Could you check a few things on this model? Use its own coordinates, in mm. A direction names the side the tool comes from. Give positions to 0.01 mm unless a question says otherwise; leave off trailing zeros. Write each loop counter-clockwise with the first axis right and the second up, starting at its lowest first coordinate (ties: lowest second). Pieces come first, ordered by that corner, then holes. Notation, with made-up numbers: (45.5, 45.25) - (74.5, 45.25) arc R23 ccw to (74.5, 61.25) - close; hole circle Ø7 at (14.25, 86). An arc over 180 degrees is marked (long way). Answer in a Markdown table with one row per item.
Autodesk Inventor part; units mm, degrees
ref_plane "YZ Plane" through (0, 0, 0) normal (1, 0, 0) x (0, 1, 0)
ref_plane "XZ Plane" through (0, 0, 0) normal (0, 1, 0) x (-1, 0, 0)
ref_plane "XY Plane" through (0, 0, 0) normal (0, 0, 1) x (1, 0, 0)
sketch "Эскиз1" plane through (0, 0, 0) normal (0, 0, 1) x (1, 0, 0)
  line L0 (0, 0) -> (12, 0)
  line L1 (12, 0) -> (12, -5)
  line L2 (12, -5) -> (0, -5)
  line L3 (0, -5) -> (0, 0)
  dimension "d0" = 12
  dimension "d1" = 5
extrude "Выдавливание1" add sketch "Эскиз1" along normal blind 5
sketch "Эскиз2" plane through (0, -5, 0) normal (0, -1, 0) x (1, 0, 0)
  line L0 (0, 0) -> (0, 5)
  line L1 (0, 0.6807) -> (2.9841, 0.6807)
  line L2 (2.9841, 0.6807) -> (2.9841, 4.0939)
  line L3 (2.9841, 4.0939) -> (4.7266, 4.0939)
  line L4 (4.7266, 4.0939) -> (4.7266, 0.6807)
  line L5 (4.7266, 0.6807) -> (5.3913, 0.6807)
  line L6 (5.3913, 0.6807) -> (5.3913, 1.8843)
  line L7 (5.3913, 1.8843) -> (7.493, 1.8843)
  line L8 (7.493, 1.8843) -> (7.493, 0.6807)
  line L9 (7.493, 0.6807) -> (7.8703, 0.6807)
  line L10 (7.8703, 0.6807) -> (7.8703, 2.8364)
  line L11 (7.8703, 2.8364) -> (8.984, 2.8364)
  line L12 (8.984, 2.8364) -> (8.984, 3.7705)
  line L13 (8.984, 3.7705) -> (9.8822, 3.7705)
  line L14 (9.8822, 3.7705) -> (9.8822, 0.6807)
  line L15 (9.8822, 0.6807) -> (11.2116, 0.6807)
  line L16 (11.2116, 0.6807) -> (11.2116, 2.5)
  line L17 (11.2116, 2.5) -> (11.517, 3.3034)
  line L18 (11.517, 3.3034) -> (12, 3.3034)
  line L19 (12, 0) -> (12, 5)
  line L20 (0, 0) -> (12, 0)
  line L21 (12, 3.3034) -> (12, 0)
  line L22 (12, 0) -> (0, 0)
  line L23 (0, 0.6807) -> (0, 3.3034)
  line L24 (0.559, 3.3034) -> (1.026, 2.5)
  line L25 (1.026, 2.5) -> (1.026, 0.6807)
  line L26 (0.559, 3.3034) -> (0, 3.3034)
extrude "Выдавливание2" cut sketch "Эскиз2" against normal blind 5 keep common part
properties part number "Преобразователь напряжения"
1) We'd pull the mould along X, two halves only. Please class faces 1 (the face through (11.362, -2.535, 2.896)), 2 (the face through (11.212, -3, 2)), 3 (the face through (0, -3, 2)), 4 (the face through (5.9, 0, 1.6)): +X half, -X half, draft (parallel to the pull), parting line (faces both ways), or undercut.
Check values:
| item | result |
|---|---|
| face 1 | undercut |
| face 2 | undercut |
| face 3 | -X half |
| face 4 | draft |
2) Imagine slicing it at C-C (x = 5). List the corners of the cut face in (y, z) for me, then the cut area to 3 significant figures.
Check values:
| item | result |
|---|---|
| outline | (-5, 0) - (0, 0) - (0, 0.68) - (-5, 0.68) - close |
| area | 3.40 mm2 |
3) Imagine slicing it at B-B (y = -2.2). List the corners of the cut face in (x, z) for me.
Check values:
| item | result |
|---|---|
| outline | (0, 0) - (12, 0) - (12, 3.3) - (11.52, 3.3) - (11.21, 2.5) - (11.21, 0.68) - (9.88, 0.68) - (9.88, 3.77) - (8.98, 3.77) - (8.98, 2.84) - (7.87, 2.84) - (7.87, 0.68) - (7.49, 0.68) - (7.49, 1.88) - (5.39, 1.88) - (5.39, 0.68) - (4.73, 0.68) - (4.73, 4.09) - (2.98, 4.09) - (2.98, 0.68) - (1.03, 0.68) - (1.03, 2.5) - (0.56, 3.3) - (0, 3.3) - close |
4) Will these pins go through, and if not, where does the flat tip stop? P1, Ø0.6, axis at x = 0.5, y = -2.5, coming from the +Z side; P2, Ø0.6, axis at x = 7, y = -2, coming from the +Z side; P3, Ø1.6, axis at x = 1.5, y = -2.5, coming from the +Z side.
Check values:
| item | result |
|---|---|
| P1 | stops at z = 3.3 |
| P2 | stops at z = 1.88 |
| P3 | stops at z = 3.06 |
5) On a 3-axis mill with a long thin cutter (end or side, diameter ignored), from which of +Z, -Z, +X, -X, +Y, -Y can I reach the whole of each face in a straight line? I mean faces 5 (the face through (4, -3, 4.094)), 6 (the face through (11, -3, 0.681)), 7 (the face through (9.4, -2.5, 3.77)). Say none if no direction works.
Check values:
| item | result |
|---|---|
| face 5 | +Z, +X, -X, +Y, -Y |
| face 6 | +Z, +Y, -Y |
| face 7 | +Z, +X, +Y, -Y |
6) If I drill on line 1 (X direction, y = -4.4, z = 2.3); line 2 (X direction, y = -0.3, z = 1.6); line 3 (Z direction, x = 9.25, y = -1.25), over which ranges is the centre line in solid material (lowest first)?
Check values:
| item | result |
|---|---|
| line 1 | x = 0 to 1.03, 2.98 to 4.73, 7.87 to 9.88, 11.21 to 12 |
| line 2 | x = 0 to 1.03, 2.98 to 4.73, 5.39 to 7.49, 7.87 to 9.88, 11.21 to 12 |
| line 3 | z = 0 to 3.77 |
7) Imagine slicing it at A-A (z = 1.5). List the corners of the cut face in (x, y) for me, then the cut area to 3 significant figures.
Check values:
| item | result |
|---|---|
| outline | (0, -5) - (1.03, -5) - (1.03, 0) - (0, 0) - close; (2.98, -5) - (4.73, -5) - (4.73, 0) - (2.98, 0) - close; (5.39, -5) - (7.49, -5) - (7.49, 0) - (5.39, 0) - close; (7.87, -5) - (9.88, -5) - (9.88, 0) - (7.87, 0) - close; (11.21, -5) - (12, -5) - (12, 0) - (11.21, 0) - close |
| area | 38.4 mm2 |
